```python
from build123d import *

# Parameters (mm, degrees)
BOSS_EXTRUDE1_DEPTH = 50
BOSS_EXTRUDE2_DEPTH = 25
CUT_EXTRUDE1_START  = -8.33
SKETCH3_R           = 22.5
CUT_EXTRUDE1_DEPTH  = 8.33
FILLET1_R           = 10
FILLET2_R           = 7
SKETCH4_R           = 10
CUT_EXTRUDE2_DEPTH  = 20


with BuildPart() as part:
    # Sketch1 → Boss-Extrude1 (new body)
    with BuildSketch(Plane.XY):
        Polygon((0, 30), (0, -30), (40, -23.334999563), (40, 23.334999563), align=None)
    extrude(amount=BOSS_EXTRUDE1_DEPTH)

    # Sketch2 → Boss-Extrude2 (add)
    with BuildSketch(Plane.XY):
        with BuildLine():
            Line((40, 0), (47.5, 0))
            ThreePointArc((47.5, 0), (48.4687848, 6.5312152), (51.291713066, 12.5))
            Line((51.291713066, 12.5), (40, 12.5))
            Line((40, 12.5), (40, 0))
        make_face()
        with BuildLine():
            Line((40, -12.5), (51.291713066, -12.5))
            ThreePointArc((51.291713066, -12.5), (48.4687848, -6.5312152), (47.5, 0))
            Line((47.5, 0), (40, 0))
            Line((40, 0), (40, -12.5))
        make_face()
        with BuildLine():
            ThreePointArc((47.5, 0), (48.4687848, -6.5312152), (51.291713066, -12.5))
            ThreePointArc((51.291713066, -12.5), (76.5312152, -21.5312152), (92.5, 0))
            Line((92.5, 0), (75, 0))
            ThreePointArc((75, 0), (70, -5), (65, 0))
            Line((65, 0), (47.5, 0))
        make_face()
        with BuildLine():
            Line((75, 0), (92.5, 0))
            ThreePointArc((92.5, 0), (76.5312152, 21.5312152), (51.291713066, 12.5))
            ThreePointArc((51.291713066, 12.5), (48.4687848, 6.5312152), (47.5, 0))
            Line((47.5, 0), (65, 0))
            ThreePointArc((65, 0), (70, 5), (75, 0))
        make_face()
    boss_extrude2 = extrude(amount=BOSS_EXTRUDE2_DEPTH)

    # Sketch3 → Cut-Extrude1 (cut)
    with BuildSketch(Plane.XY.offset(25).offset(CUT_EXTRUDE1_START)):
        with Locations((70, 0)):
            Circle(SKETCH3_R)
    cut_extrude1 = extrude(amount=CUT_EXTRUDE1_DEPTH, mode=Mode.SUBTRACT)

    # Mirror1: Boss-Extrude2, Cut-Extrude1 across plane
    add(boss_extrude2.mirror(Plane.XY.offset(25)))
    add(cut_extrude1.mirror(Plane.XY.offset(25)), mode=Mode.SUBTRACT)

    # Fillet1
    fillet1_edges = [part.edges().sort_by_distance(p)[0] for p in [
        (51.291713066, 12.5, 8.335),
        (51.291713066, -12.5, 8.335),
        (51.291713066, -12.5, 41.665),
        (51.291713066, 12.5, 41.665),
    ]]
    fillet(fillet1_edges, radius=FILLET1_R)

    # Fillet2
    fillet2_edges = [part.edges().sort_by_distance(p)[0] for p in [
        (40, 23.334999563, 25),
        (40, -23.334999563, 25),
    ]]
    fillet(fillet2_edges, radius=FILLET2_R)

    # Sketch4 → Cut-Extrude2 (cut)
    with BuildSketch(Plane.ZY):
        with Locations((25, 0)):
            Circle(SKETCH4_R)
    extrude(amount=-CUT_EXTRUDE2_DEPTH, mode=Mode.SUBTRACT)


solid = part.part
```
Work out the finished part from the listing and answer in its coordinate system (mm). A direction names the side the tool comes from. Coordinates: 2 decimals unless noted, no trailing zeros. Order: outer loops, then holes, each group sorted by start corner. A loop starts at its lowest first (then second) coordinate and runs counter-clockwise, first axis right, second up. Notation, with made-up numbers: M 43.25,42 L 66.25,42 A18 cw 66.25,70 Z; hole C 6,30.25 d3. An arc over 180 degrees is marked long. Use CSV: the item, a comma, the result in double quotes.
1) Section A-A on x = 70 is taken. Write down the section's boundary in (y, z).
Worked out:
outline,"M -22.5,0 L -5,0 L -5,16.67 L -22.5,16.67 Z; M -22.5,33.33 L -5,33.33 L -5,50 L -22.5,50 Z; M 5,0 L 22.5,0 L 22.5,16.67 L 5,16.67 Z; M 5,33.33 L 22.5,33.33 L 22.5,50 L 5,50 Z"
2) For faces 1 (the face through (50.522, 13.324, 8.452)), 2 (the face through (44, 12.5, 25)), 3 (the face through (38.385, -21.877, 25.35)), 4 (the face through (17.314, 27.115, 24.65)), 5 (the face through (20, 0, 25)), determine the directions among +Z, -Z, +X, -X, +Y, -Y from which every point of the face is accessible in a straight line to the end or side of a thin tool.
Worked out:
face 1,"+Z, -Z, +Y"
face 2,"+Y"
face 3,"+Z, -Z, -Y"
face 4,"+Z, -Z, +X, +Y"
face 5,"-X"
3) Section C-C on z = 9 is taken. Write down the section's boundary in (x, y), plus the area to 3 significant figures.
Worked out:
outline,"M 0,-30 L 34.15,-24.31 A7 ccw 40,-17.4 L 40,-12.5 L 46.55,-12.5 A10 cw 53.76,-15.58 A22.5 ccw long 53.76,15.58 A10 cw 46.55,12.5 L 40,12.5 L 40,17.4 A7 ccw 34.15,24.31 L 0,30 Z; hole C 70,0 d10"
area,"3,850 mm^2"
4) Section B-B on y = -1.5 is taken. Write down the section's boundary in (x, z), plus the area to 3 significant figures.
Worked out:
outline,"M 0,0 L 65.23,0 L 65.23,16.67 L 47.55,16.67 L 47.55,33.33 L 65.23,33.33 L 65.23,50 L 0,50 L 0,34.89 L 20,34.89 L 20,15.11 L 0,15.11 Z; M 74.77,0 L 92.45,0 L 92.45,16.67 L 74.77,16.67 Z; M 74.77,33.33 L 92.45,33.33 L 92.45,50 L 74.77,50 Z"
area,"3,160 mm^2"
5) Determine the mould class of faces 6 (the face through (9.86, 3, 34.54)), 7 (the face through (40, 15, 25)), 8 (the face through (50.42, 13.28, 41.55)), 9 (the face through (47.5, 0.2, 25.1)) for opening direction X: released by +X, released by -X, zero draft, split by the parting line, or undercut.
Worked out:
face 6,"zero draft"
face 7,"undercut"
face 8,"undercut"
face 9,"released by +X"
6) Consider line 1 (Z direction, x = 63, y = 14); line 2 (X direction, y = 0, z = 5.5); line 3 (Y direction, x = 70, z = 6). Determine where each line is inside the solid, lowest interval first. Write a range as [from, to].
Worked out:
line 1,"z = [0, 16.67], [33.33, 50]"
line 2,"x = [0, 65], [75, 92.5]"
line 3,"y = [-22.5, -5], [5, 22.5]"
7) Section D-D on z = 25 is taken. Write down the section's boundary in (x, y), plus the area to 3 significant figures.
Worked out:
outline,"M 0,-30 L 34.15,-24.31 A7 ccw 40,-17.4 L 40,-12.5 L 51.29,-12.5 A22.5 cw 51.29,12.5 L 40,12.5 L 40,17.4 A7 ccw 34.15,24.31 L 0,30 L 0,10 L 20,10 L 20,-10 L 0,-10 Z"
area,"1,940 mm^2"
8) Flat-ended cylindrical pins translate along their axes: pin 1 Ø5 at (y, z) = (-17, 44.5) entering from +X; pin 2 Ø12.5 at (x, z) = (44, 29) entering from -Y; pin 3 Ø1.5 at (y, z) = (14, 23) entering from +X. Find the tip coordinate at first contact, or state that the pin passes through.
Worked out:
pin 1,"stops at x = 87.2"
pin 2,"stops at y = -22.55"
pin 3,"stops at x = 40"
